from build123d import *

# Parameters (mm, degrees)
SKETCH1_W               = 108.761980125
SKETCH1_H               = 61.936744186
BOSS_EXTRUDE1_DEPTH     = 2
SKETCH2_R               = 2.4
CUT_EXTRUDE1_DEPTH      = 63.943741049
MIRROR2_COPY_1_SKETCH_R = 2.4
MIRROR2_COPY_1_DEPTH    = 63.943741049
SKETCH3_W               = 94.024869854
SKETCH3_H               = 56.555498618
CUT_EXTRUDE2_DEPTH      = 63.943741049
SKETCH6_W               = 101.2762547
SKETCH6_H               = 61.936744186
CUT_EXTRUDE5_DEPTH      = 10
SKETCH8_W               = 0.808555921
SKETCH8_H               = 61.936744186
BOSS_EXTRUDE2_DEPTH     = 8
SKETCH10_W              = 8.294281346
SKETCH10_H              = 61.936744186
BOSS_EXTRUDE4_DEPTH     = 1
CUT_EXTRUDE6_START      = -0.5
SKETCH11_R              = 2.4
CUT_EXTRUDE6_DEPTH      = 0.5


with BuildPart() as part:
    # Sketch1 → Boss-Extrude1 (new body)
    with BuildSketch(Plane(origin=(0, 0, 0), x_dir=(1, 0, 0), z_dir=(0, 1, 0))):
        with Locations((-0.380990063, 0)):
            Rectangle(SKETCH1_W, SKETCH1_H)
    extrude(amount=BOSS_EXTRUDE1_DEPTH)

    # Sketch2 → Cut-Extrude1 (cut, symmetric)
    with BuildSketch(Plane(origin=(0, 2, 0), x_dir=(1, 0, 0), z_dir=(0, 1, 0))):
        with Locations(Location((-50.814865351, 26.477784527, 0), (0, 0, 270))):
            Circle(SKETCH2_R)
    cut_extrude1 = extrude(amount=CUT_EXTRUDE1_DEPTH, both=True, mode=Mode.SUBTRACT)

    # Mirror1: Cut-Extrude1 across plane
    add(cut_extrude1.mirror(Plane.XY), mode=Mode.SUBTRACT)

    # Mirror2: Cut-Extrude1 across plane
    add(cut_extrude1.mirror(Plane.ZY.offset(0.380990062)), mode=Mode.SUBTRACT)

    # Mirror2 copy 1 sketch → Mirror2 copy 1 (cut, symmetric)
    with BuildSketch(Plane(origin=(-0.761980125, 2, 0), x_dir=(-1, 0, 0), z_dir=(0, 1, 0))):
        with Locations(Location((-50.814865351, 26.477784527, 0), (0, 0, 270))):
            Circle(MIRROR2_COPY_1_SKETCH_R)
    extrude(amount=MIRROR2_COPY_1_DEPTH, both=True, mode=Mode.SUBTRACT)

    # Sketch3 → Cut-Extrude2 (cut, through all)
    with BuildSketch(Plane(origin=(0, 2, 0), x_dir=(1, 0, 0), z_dir=(0, 1, 0))):
        Rectangle(SKETCH3_W, SKETCH3_H)
    extrude(amount=-CUT_EXTRUDE2_DEPTH, mode=Mode.SUBTRACT)

    # Sketch6 → Cut-Extrude5 (cut)
    with BuildSketch(Plane(origin=(0, 2, 0), x_dir=(1, 0, 0), z_dir=(0, 1, 0))):
        with Locations((3.36187265, 0)):
            Rectangle(SKETCH6_W, SKETCH6_H)
    extrude(amount=-CUT_EXTRUDE5_DEPTH, mode=Mode.SUBTRACT)

    # Sketch8 → Boss-Extrude2 (add)
    with BuildSketch(Plane(origin=(0, 2, 0), x_dir=(1, 0, 0), z_dir=(0, 1, 0))):
        with Locations((-55.166258086, 0)):
            Rectangle(SKETCH8_W, SKETCH8_H)
    extrude(amount=-BOSS_EXTRUDE2_DEPTH)

    # Sketch10 → Boss-Extrude4 (add)
    with BuildSketch(Plane(origin=(0, 2, 0), x_dir=(1, 0, 0), z_dir=(0, 1, 0))):
        with Locations((-51.423395373, 0)):
            Rectangle(SKETCH10_W, SKETCH10_H)
    extrude(amount=BOSS_EXTRUDE4_DEPTH)

    # Sketch11 → Cut-Extrude6 (cut)
    with BuildSketch(Plane.XZ.offset(-2).offset(CUT_EXTRUDE6_START)):
        with Locations(Location((-50.814865351, -26.477784527, 0), (0, 0, 90))):
            Circle(SKETCH11_R)
        with Locations(Location((-50.814865351, 26.477784527, 0), (0, 0, 270))):
            Circle(SKETCH11_R)
    extrude(amount=CUT_EXTRUDE6_DEPTH, mode=Mode.SUBTRACT)


solid = part.part
Design review of the part built by this model. Coordinates are the model's own, in mm. A direction names the side the tool comes from. Give positions to 0.01 mm unless a question says otherwise; leave off trailing zeros. Loops run counter-clockwise (first coordinate to the right, second up) from the corner with the lowest first, then second, coordinate; pieces in that order, holes last. Notation, with made-up numbers: (64.25, 71.25) - (105.25, 71.25) arc R22 cw to (105.25, 83.25) - close; hole circle Ø3 at (59.25, 2.25). An arc over 180 degrees is marked (long way). Use CSV: the item, a comma, the result in double quotes. Start each with the question number.
1. Draft analysis for pull direction X (two halves, no side actions). For faces 4 (the cylindrical face through (-48.435, 1.268, 26.79)), 5 (the flat face through (-55.571, -2, 0)), 6 (the flat face through (-51, 0, 0)), state which applies: released by +X, released by -X, zero draft, split by the parting line, or undercut.
2. Add section B-B (y = -2.75). State the section outline as (x, z) points, plus the area to 3 significant figures.
3. Machinability: for faces 1 (the flat face through (-51, 2.5, 27)), 2 (the flat face through (-52.4, 0.4, -30.968)), 3 (the flat face through (-54.762, -3, 0)), which of the approach directions +Z, -Z, +X, -X, +Y, -Y give a long, thin tool a straight path to every point of the face, cutting with its end or side? Answer none if there is none.
4. Add section C-C (z = -14.5). State the section outline as (x, y) points, plus the area to 3 significant figures.
5. Insertion check: P1, Ø3.5, axis at x = -49, z = 1.5, coming from the -Y side; P2, Ø1.4, axis at x = -50, z = -25.5, coming from the -Y side. Each pin has a flat end and moves straight along its axis. Give the tip position at first contact, or say it passes through.
6. Add section D-D (x = -51.75). State the section outline as (y, z) points, plus the area to 3 significant figures.
7. Add section A-A (x = -49.5). State the section outline as (y, z) points.
8. Wall thickness on L1, parallel to Y at x = -48, z = -12.5; L2, parallel to X at y = -2, z = -21; L3, parallel to Y at x = -52.5, z = -25: over which ranges is each line inside the solid? List them lowest first.
Results found:
1,face 4,"undercut"
1,face 5,"released by -X"
1,face 6,"zero draft"
2,outline,"(-55.57, -30.97) - (-54.76, -30.97) - (-54.76, 30.97) - (-55.57, 30.97) - close"
2,area,"50.1 mm²"
3,face 1,"-Y"
3,face 2,"-Z, +X, -X, +Y, -Y"
3,face 3,"+Z, -Z, +X, -Y"
4,outline,"(-55.57, -6) - (-54.76, -6) - (-54.76, 0) - (-47.28, 0) - (-47.28, 3) - (-55.57, 3) - close"
4,area,"29.7 mm²"
5,P1,"stops at y = 0"
5,P2,"stops at y = 2.5"
6,outline,"(0, -30.97) - (3, -30.97) - (3, 30.97) - (0, 30.97) - (0, 28.69) - (2.5, 28.69) - (2.5, 24.27) - (0, 24.27) - (0, -24.27) - (2.5, -24.27) - (2.5, -28.69) - (0, -28.69) - close"
6,area,"164 mm²"
7,outline,"(0, -30.97) - (3, -30.97) - (3, 30.97) - (0, 30.97) - (0, 28.49) - (2.5, 28.49) - (2.5, 24.47) - (0, 24.47) - (0, -24.47) - (2.5, -24.47) - (2.5, -28.49) - (0, -28.49) - close"
8,L1,"y = 0 to 3"
8,L2,"x = -55.57 to -54.76"
8,L3,"y = 2.5 to 3"
